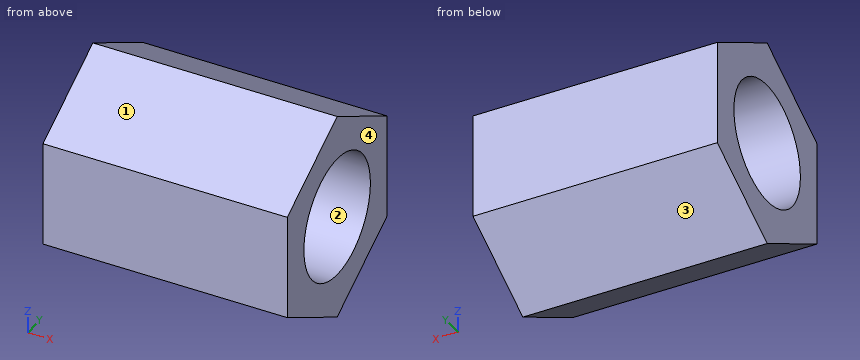
```python
from build123d import *

# Parameters (mm, degrees)
SKETCH_1_R          = 1.5
EXTRUDE_1_DEPTH     = 6
EXTRUDE_2_DEPTH     = 6
CUT_EXTRUDE_START   = -7
SKETCH_4_R          = 1.5
CUT_EXTRUDE_1_DEPTH = 7
SKETCH_5_R          = 2.902740869
CUT_EXTRUDE_2_DEPTH = 6


with BuildPart() as part:
    # 草图1 → 凸台-拉伸1 (new body)
    with BuildSketch(Plane(origin=(0, 0, 0), x_dir=(0, 0, -1), z_dir=(1, 0, 0))):
        Circle(SKETCH_1_R)
    extrude(amount=EXTRUDE_1_DEPTH)

    # 草图2 → 凸台-拉伸2 (add)
    with BuildSketch(Plane(origin=(6, 0, 0), x_dir=(0, 0, -1), z_dir=(1, 0, 0))):
        Polygon((2.598076211, 0), (1.299038106, 2.25), (-1.299038106, 2.25), (-2.598076211, 0), (-1.299038106, -2.25), (1.299038106, -2.25), align=None)
    extrude(amount=EXTRUDE_2_DEPTH)

    # 草图4 → 切除-拉伸1 (cut)
    with BuildSketch(Plane(origin=(12, 0, 0), x_dir=(0, 0, -1), z_dir=(1, 0, 0)).offset(CUT_EXTRUDE_START)):
        Circle(SKETCH_4_R)
    extrude(amount=CUT_EXTRUDE_1_DEPTH, mode=Mode.SUBTRACT)


with BuildPart() as cut_extrude_1_piece_1:
    # of the separate pieces the step leaves, piece 1, a body of its own (cut_extrude_1_pieces)
    add(part.part.solids().sort_by_distance((6, 0, -2.598076211))[0])


with BuildPart() as cut_extrude_1_piece_2:
    # of the separate pieces the step leaves, piece 2, a body of its own (cut_extrude_1_pieces)
    add(part.part.solids().sort_by_distance((0, 0, -1.5))[0])

    # 草图5 → 切除-拉伸2 (cut)
    with BuildSketch(Plane.ZY):
        Circle(SKETCH_5_R)
    extrude(amount=-CUT_EXTRUDE_2_DEPTH, mode=Mode.SUBTRACT)


solid = cut_extrude_1_piece_1.part
```
Geometry check sheet. Reference: the model listing, model coordinates, mm. Face numbers are marked on the shaded views. Coordinates: 2 decimals unless noted, no trailing zeros. Loops run counter-clockwise (first coordinate to the right, second up) from the corner with the lowest first, then second, coordinate; pieces in that order, holes last.
Item 1: Sectioned sample at D-D, the plane z = 2.1. Record the boundary of the cut face in (x, y).
Item 2: Release check for a two-part mould opening along Z. For the marked faces 1, 2, 3 and 4 record: released by +Z, released by -Z, zero draft, split by the parting line, or undercut.
Item 3: Thickness scan on line 1 (Y direction, x = 8.6, z = 0); line 2 (Y direction, x = 7.5, z = 1.1); line 3 (Z direction, x = 9.85, y = 0.8). Record the ranges inside material, lowest first.
Item 4: Sectioned sample at B-B, the plane y = 0.5. Record the boundary of the cut face in (x, z).
Item 5: Sectioned sample at A-A, the plane x = 8.6. Record the boundary of the cut face in (y, z), then the cut area to 3 significant figures.
Item 6: Go/stop test with flat-tipped pins: pin 1 Ø2 at (x, y) = (10.5, 0.5) entering from -Z; pin 2 Ø1.5 at (x, y) = (8.5, -1) entering from -Z. Record where each tip stops, or that it passes through.
Item 7: Sectioned sample at C-C, the plane z = -0.8. Record the boundary of the cut face in (x, y), then the cut area to 3 significant figures.
Check result:
1. outline: (6, -0.86) - (12, -0.86) - (12, 0.86) - (6, 0.86) - close
2. face 1: released by +Z
2. face 2: undercut
2. face 3: released by -Z
2. face 4: zero draft
3. line 1: y = -2.25 to -1.5, 1.5 to 2.25
3. line 2: y = -2.25 to -1.02, 1.02 to 2.25
3. line 3: z = -2.14 to -1.27, 1.27 to 2.14
4. outline: (6, -2.31) - (12, -2.31) - (12, -1.41) - (6, -1.41) - close; (6, 1.41) - (12, 1.41) - (12, 2.31) - (6, 2.31) - close
5. outline: (-2.25, -1.3) - (0, -2.6) - (2.25, -1.3) - (2.25, 1.3) - (0, 2.6) - (-2.25, 1.3) - close; hole circle Ø3 at (0, 0)
5. area: 10.5 mm2
6. pin 1: stops at z = -2.6
6. pin 2: stops at z = -2.45
7. outline: (6, -2.25) - (12, -2.25) - (12, -1.27) - (6, -1.27) - close; (6, 1.27) - (12, 1.27) - (12, 2.25) - (6, 2.25) - close
7. area: 11.8 mm2
